Here's how the part is built. I have some questions about the finished solid (model axes, mm). A direction names the side the tool comes from. Coordinates: 2 decimals unless noted, no trailing zeros. Write each loop counter-clockwise with the first axis right and the second up, starting at its lowest first coordinate (ties: lowest second). Pieces come first, ordered by that corner, then holes. Notation, with made-up numbers: (88, 15.5) -> (95, 15.5) arc R24 ccw to (95, 48.5) -> close; hole circle Ø6 at (57.5, -17.5). An arc over 180 degrees is marked (long way). Put each result on its own line as item: value. Start each with the question number.
Item 1: I need wall thicknesses on line 1 (Z direction, x = 520.7, y = -168); line 2 (Z direction, x = -520, y = -374); line 3 (X direction, y = -487, z = 215). Which ranges of each line are inside material? Lowest first, please. Write a range as [from, to].
Item 2: For pin 1 (19 mm diameter, centred on x = -513, z = 200.5, fed in from -Y); pin 2 (12 mm diameter, centred on y = -365.5, z = 181, fed in from +X); pin 3 (12 mm diameter, centred on x = 427.5, z = 208.5, fed in from -Y), each with a flat end and sliding along its axis, tell me the tip position at first contact or that it passes through.
Item 3: I want a section at D-D, the plane z = 102.5. List the corners of the cut face in (x, y) for me.
Item 4: On a 3-axis mill with a long thin cutter (end or side, diameter ignored), from which of +Z, -Z, +X, -X, +Y, -Y can I reach the whole of each face in a straight line? I mean faces 1 (the face through (516.57, -346.99, -184.42)), 2 (the face through (-521, -635, -248)). Say none if no direction works.
Item 5: I want a section at B-B, the plane z = 215.9. List the corners of the cut face in (x, y) for me, then the cut area to 3 significant figures.
Item 6: I want a section at C-C, the plane x = -520.7. List the corners of the cut face in (y, z) for me.
Item 7: If we mould it in two halves opening along Z, with no side actions, what happens to faces 3 (the face through (506, -635, -187)), 4 (the face through (-9, 0, -4))? For each: released by +Z, released by -Z, zero draft, split by the parting line, or undercut.
Item 8: I want a section at A-A, the plane y = -224.5. List the corners of the cut face in (x, z) for me, then the cut area to 3 significant figures.
from build123d import *

# Parameters (mm, degrees)
SKETCH1_W           = 1219.2
SKETCH1_H           = 609.6
BOSS_EXTRUDE1_DEPTH = 19.05
SKETCH2_R           = 63.5
BOSS_EXTRUDE2_DEPTH = 25.4
SKETCH3_R           = 38.1
SKETCH3_R_2         = 36.165456998
BOSS_EXTRUDE3_DEPTH = 609.6
SKETCH4_R           = 31.75
CUT_EXTRUDE1_DEPTH  = 584.2


with BuildPart() as part:
    # Sketch1 → Boss-Extrude1 (new body)
    with BuildSketch(Plane(origin=(0, 0, 0), x_dir=(1, 0, 0), z_dir=(0, 1, 0))):
        Rectangle(SKETCH1_W, SKETCH1_H)
    extrude(amount=BOSS_EXTRUDE1_DEPTH)

    # Sketch2 → Boss-Extrude2 (add)
    with BuildSketch(Plane.XZ):
        with Locations((-520.7, 215.9)):
            Circle(SKETCH2_R)
        with Locations((-520.7, -215.9)):
            Circle(SKETCH2_R)
        with Locations((520.7, 215.9)):
            Circle(SKETCH2_R)
        with Locations((520.7, -215.9)):
            Circle(SKETCH2_R)
    extrude(amount=BOSS_EXTRUDE2_DEPTH)

    # Sketch3 → Boss-Extrude3 (add)
    with BuildSketch(Plane.XZ.offset(25.4)):
        with Locations((-520.7, 215.9)):
            Circle(SKETCH3_R)
        with Locations((-520.7, -215.9)):
            Circle(SKETCH3_R_2)
        with Locations((520.7, 215.9)):
            Circle(SKETCH3_R)
        with Locations((520.7, -215.9)):
            Circle(SKETCH3_R)
    extrude(amount=BOSS_EXTRUDE3_DEPTH)

    # Sketch4 → Cut-Extrude1 (cut)
    with BuildSketch(Plane.XZ.offset(635)):
        with Locations((-520.7, 215.9)):
            Circle(SKETCH4_R)
        with Locations((520.7, 215.9)):
            Circle(SKETCH4_R)
        with Locations((520.7, -215.9)):
            Circle(SKETCH4_R)
        with Locations((-520.7, -215.9)):
            Circle(SKETCH4_R)
    extrude(amount=-CUT_EXTRUDE1_DEPTH, mode=Mode.SUBTRACT)


solid = part.part
Calculated:
1. line 1: z = [-254, -247.65], [-184.15, -177.8], [177.8, 184.15], [247.65, 254]
1. line 2: z = [-252.06, -247.64], [-184.16, -179.74], [177.81, 184.16], [247.64, 253.99]
1. line 3: x = [-558.79, -552.44], [-488.96, -482.61], [482.61, 488.96], [552.44, 558.79]
2. pin 1: stops at y = -50.8
2. pin 2: stops at x = 545.53
2. pin 3: stops at y = 0
3. outline: (-609.6, 0) -> (609.6, 0) -> (609.6, 19.05) -> (-609.6, 19.05) -> close
4. face 1: -Y
4. face 2: +Z, -Z, +X, -X, -Y
5. outline: (-609.6, 0) -> (-584.2, 0) -> (-584.2, -25.4) -> (-558.8, -25.4) -> (-558.8, -635) -> (-552.45, -635) -> (-552.45, -50.8) -> (-488.95, -50.8) -> (-488.95, -635) -> (-482.6, -635) -> (-482.6, -25.4) -> (-457.2, -25.4) -> (-457.2, 0) -> (457.2, 0) -> (457.2, -25.4) -> (482.6, -25.4) -> (482.6, -635) -> (488.95, -635) -> (488.95, -50.8) -> (552.45, -50.8) -> (552.45, -635) -> (558.8, -635) -> (558.8, -25.4) -> (584.2, -25.4) -> (584.2, 0) -> (609.6, 0) -> (609.6, 19.05) -> (-609.6, 19.05) -> close
5. area: 48,400 mm2
6. outline: (-635, -252.07) -> (-25.4, -252.07) -> (-25.4, -279.4) -> (0, -279.4) -> (0, -304.8) -> (19.05, -304.8) -> (19.05, 304.8) -> (0, 304.8) -> (0, 279.4) -> (-25.4, 279.4) -> (-25.4, 254) -> (-635, 254) -> (-635, 247.65) -> (-50.8, 247.65) -> (-50.8, 184.15) -> (-635, 184.15) -> (-635, 177.8) -> (-25.4, 177.8) -> (-25.4, 152.4) -> (0, 152.4) -> (0, -152.4) -> (-25.4, -152.4) -> (-25.4, -179.73) -> (-635, -179.73) -> (-635, -184.15) -> (-50.8, -184.15) -> (-50.8, -247.65) -> (-635, -247.65) -> close
7. face 3: zero draft
7. face 4: undercut
8. outline: circle Ø76.2 at (-520.7, 215.9); circle Ø72.33 at (-520.7, -215.9); circle Ø76.2 at (520.7, -215.9); circle Ø76.2 at (520.7, 215.9); hole circle Ø63.5 at (-520.7, -215.9); hole circle Ø63.5 at (-520.7, 215.9); hole circle Ø63.5 at (520.7, -215.9); hole circle Ø63.5 at (520.7, 215.9)
8. area: 5,120 mm2
